from build123d import *

# Parameters (mm, degrees)
SKETCH1_R           = 2.25
SKETCH1_R_2         = 2
SKETCH1_W           = 13.333333333
SKETCH1_H           = 3.675
SKETCH1_W_2         = 13.333333334
SKETCH1_W_3         = 3.675
SKETCH1_H_2         = 11.818181818
BOSS_EXTRUDE1_DEPTH = 6.35


with BuildPart() as part:
    # Sketch1 → Boss-Extrude1 (new body)
    with BuildSketch(Plane.XY):
        with BuildLine():
            Line((-54.514802885, -31.577464534), (54.514802885, -31.577464534))
            ThreePointArc((54.514802885, -31.577464534), (0, 63), (-54.514802885, -31.577464534))
        make_face()
        with Locations((-51.25, 23.184046239)):
            Circle(SKETCH1_R, mode=Mode.SUBTRACT)
        with Locations((-51.25, -12.496398734)):
            Circle(SKETCH1_R, mode=Mode.SUBTRACT)
        with Locations((-30.629163068, 48.823601552)):
            Circle(SKETCH1_R_2, mode=Mode.SUBTRACT)
        with Locations((51.25, 23.184046239)):
            Circle(SKETCH1_R, mode=Mode.SUBTRACT)
        with Locations((51.25, -12.496398734)):
            Circle(SKETCH1_R, mode=Mode.SUBTRACT)
        with Locations((-19.525679125, 38.728601552)):
            Circle(SKETCH1_R_2, mode=Mode.SUBTRACT)
        with Locations((-19.525679125, -18.421398448)):
            Circle(SKETCH1_R_2, mode=Mode.SUBTRACT)
        with Locations((19.844320875, -18.421398448)):
            Circle(SKETCH1_R_2, mode=Mode.SUBTRACT)
        with Locations((19.844320875, 38.728601552)):
            Circle(SKETCH1_R_2, mode=Mode.SUBTRACT)
        with Locations((26.666666666, -26.564964534)):
            Rectangle(SKETCH1_W, SKETCH1_H, mode=Mode.SUBTRACT)
        with Locations((0, -26.564964534)):
            Rectangle(SKETCH1_W_2, SKETCH1_H, mode=Mode.SUBTRACT)
        with Locations((-26.666666666, -26.564964534)):
            Rectangle(SKETCH1_W, SKETCH1_H, mode=Mode.SUBTRACT)
        with Locations((-41.8375, -12.909282716)):
            Rectangle(SKETCH1_W_3, SKETCH1_H_2, mode=Mode.SUBTRACT)
        with Locations((-41.8375, 10.727080921)):
            Rectangle(SKETCH1_W_3, SKETCH1_H_2, mode=Mode.SUBTRACT)
        with Locations((-41.8375, 34.363444557)):
            Rectangle(SKETCH1_W_3, SKETCH1_H_2, mode=Mode.SUBTRACT)
        with Locations((41.8375, -12.909282716)):
            Rectangle(SKETCH1_W_3, SKETCH1_H_2, mode=Mode.SUBTRACT)
        with Locations((41.8375, 10.727080921)):
            Rectangle(SKETCH1_W_3, SKETCH1_H_2, mode=Mode.SUBTRACT)
        with Locations((41.8375, 34.363444557)):
            Rectangle(SKETCH1_W_3, SKETCH1_H_2, mode=Mode.SUBTRACT)
        with BuildLine():
            Line((25.265, 44.378601552), (25.265, 53.268601552))
            ThreePointArc((25.265, 53.268601552), (25.118553391, 53.622154943), (24.765, 53.768601552))
            Line((24.765, 53.768601552), (-24.765, 53.768601552))
            ThreePointArc((-24.765, 53.768601552), (-25.118553391, 53.622154943), (-25.265, 53.268601552))
            Line((-25.265, 53.268601552), (-25.265, 44.378601552))
            ThreePointArc((-25.265, 44.378601552), (-25.118553391, 44.025048162), (-24.765, 43.878601552))
            Line((-24.765, 43.878601552), (24.765, 43.878601552))
            ThreePointArc((24.765, 43.878601552), (25.118553391, 44.025048162), (25.265, 44.378601552))
        make_face(mode=Mode.SUBTRACT)
    extrude(amount=-BOSS_EXTRUDE1_DEPTH)


solid = part.part
CAD build for the part. Positions are in the model's coordinates, mm. A direction names the side the tool comes from. Round coordinates to 2 decimals unless told otherwise and drop trailing zeros. Loops run counter-clockwise (first coordinate to the right, second up) from the corner with the lowest first, then second, coordinate; pieces in that order, holes last. Notation, with made-up numbers: M 54.25,59 L 66.25,59 A13 cw 66.25,83 Z; hole C 9.5,-29 d7. An arc over 180 degrees is marked long. One line per question, with ' | ' between items. Start each with the question number.
Item 1: Cut at B-B, the plane x = -15.5. Write the cut outline in (y, z), plus the area to 3 significant figures.
Item 2: Cut at A-A, the plane x = 0. Write the cut outline in (y, z), plus the area to 3 significant figures.
Item 3: Cut at C-C, the plane y = 32.5. Write the cut outline in (x, z) (3 decimals), plus the area to 3 significant figures.
Item 4: Wall check: line 1 (Y direction, x = -0.5, z = -1.75); line 2 (X direction, y = 15, z = -1) (3 decimals); line 3 (Y direction, x = -3.5, z = -1.25). Give the ranges that are in metal, low to high.
Item 5: Pin check, flat tips, straight feed: pin 1 Ø1 at (x, z) = (4.5, -2.5) entering from +Y; pin 2 Ø1.1 at (y, z) = (-27, -3.5) entering from +X; pin 3 Ø1.5 at (y, z) = (14, -4.5) entering from +X. Stop position of each tip, or through.
Item 6: Which spindle directions (+Z, -Z, +X, -X, +Y, -Y) get a long thin tool onto all of the face, cutting with end or side? Do faces 1 (the flat face through (-1, 6, 0)), 2 (the flat face through (-25.265, 49, -3)). Say none if no direction does.
Item 7: Cut at D-D, the plane x = 14.5. Write the cut outline in (y, z), plus the area to 3 significant figures.
Responses:
1) outline: M -31.58,-6.35 L 43.88,-6.35 L 43.88,0 L -31.58,0 Z; M 53.77,-6.35 L 61.06,-6.35 L 61.06,0 L 53.77,0 Z | area: 525 mm²
2) outline: M -31.58,-6.35 L -28.4,-6.35 L -28.4,0 L -31.58,0 Z; M -24.73,-6.35 L 43.88,-6.35 L 43.88,0 L -24.73,0 Z; M 53.77,-6.35 L 63,-6.35 L 63,0 L 53.77,0 Z | area: 514 mm²
3) outline: M -53.97,-6.35 L -43.675,-6.35 L -43.675,0 L -53.97,0 Z; M -40,-6.35 L 40,-6.35 L 40,0 L -40,0 Z; M 43.675,-6.35 L 53.97,-6.35 L 53.97,0 L 43.675,0 Z | area: 639 mm²
4) line 1: y = -31.58 to -28.4, -24.73 to 43.88, 53.77 to 63 | line 2: x = -61.188 to -43.675, -40 to 40, 43.675 to 61.188 | line 3: y = -31.58 to -28.4, -24.73 to 43.88, 53.77 to 62.9
5) pin 1: stops at y = 62.87 | pin 2: stops at x = 57.18 | pin 3: stops at x = 61.59
6) face 1: +Z, +X, -X, +Y, -Y | face 2: +Z, -Z
7) outline: M -31.58,-6.35 L 43.88,-6.35 L 43.88,0 L -31.58,0 Z; M 53.77,-6.35 L 61.31,-6.35 L 61.31,0 L 53.77,0 Z | area: 527 mm²
